Can you work these out from the model? Positions are in its coordinate system, mm. Coordinates: 2 decimals unless noted, no trailing zeros. Order: outer loops, then holes, each group sorted by start corner. A loop starts at its lowest first (then second) coordinate and runs counter-clockwise, first axis right, second up. Notation, with made-up numbers: (-12, -39.5) -> (28, -39.5) arc R22 cw to (28, -18.5) -> close; hole circle Ø5 at (-16, -15). An arc over 180 degrees is marked (long way). Answer in a Markdown table with one row per item.
```python
from build123d import *

# Parameters (mm, degrees)
SKETCH_1_W      = 74
SKETCH_1_H      = 105
SKETCH_1_R      = 2.1
EXTRUDE_1_DEPTH = 3
FILLET_1_R      = 5
CHAMFER_1_SIZE  = 1.5


with BuildPart() as part:
    # ｽｹｯﾁ1 → ﾎﾞｽ - 押し出し1 (new body)
    with BuildSketch(Plane.XY):
        Rectangle(SKETCH_1_W, SKETCH_1_H)
        with Locations((-16, 36)):
            Circle(SKETCH_1_R, mode=Mode.SUBTRACT)
        with Locations((16, 36)):
            Circle(SKETCH_1_R, mode=Mode.SUBTRACT)
        with Locations((-16, 4)):
            Circle(SKETCH_1_R, mode=Mode.SUBTRACT)
        with Locations((16, 4)):
            Circle(SKETCH_1_R, mode=Mode.SUBTRACT)
        with Locations((-29.5, 45)):
            Circle(SKETCH_1_R, mode=Mode.SUBTRACT)
        with Locations((-29.5, -45)):
            Circle(SKETCH_1_R, mode=Mode.SUBTRACT)
        with Locations((29.5, 45)):
            Circle(SKETCH_1_R, mode=Mode.SUBTRACT)
        with Locations((29.5, -45)):
            Circle(SKETCH_1_R, mode=Mode.SUBTRACT)
    extrude(amount=EXTRUDE_1_DEPTH)

    # ﾌｨﾚｯﾄ1
    fillet_1_edges = [part.edges().sort_by_distance(p)[0] for p in [
        (37, -52.5, 1.5),
        (-37, -52.5, 1.5),
        (-37, 52.5, 1.5),
        (37, 52.5, 1.5),
    ]]
    fillet(fillet_1_edges, radius=FILLET_1_R)

    # 面取り1
    chamfer_1_edges = [part.edges().sort_by_distance(p)[0] for p in [
        (-18.1, 36, 3),
        (13.9, 36, 3),
        (-18.1, 4, 3),
        (13.9, 4, 3),
    ]]
    chamfer(chamfer_1_edges, length=CHAMFER_1_SIZE)


solid = part.part
```
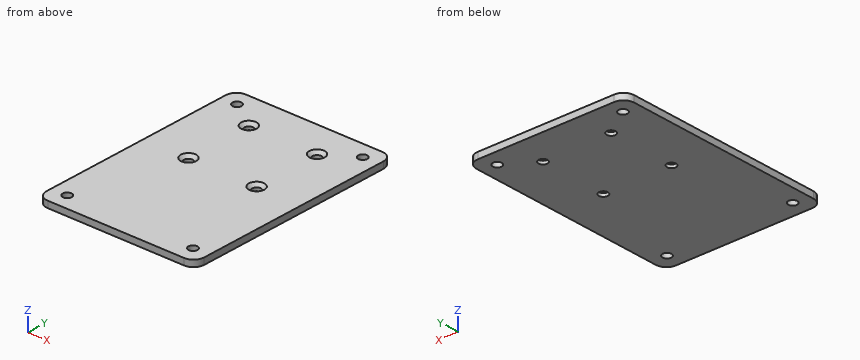
(1) Will this pin go through, and if not, where does the flat tip stop? pin 1 Ø4 at (x, y) = (-16, 36) entering from -Z.
Response values:
| item | result |
|---|---|
| pin 1 | through |
(2) I need wall thicknesses on line 1 (Y direction, x = 29.5, z = 1.4); line 2 (Y direction, x = 18, z = 1.85); line 3 (X direction, y = 44, z = 0.55). Which ranges of each line are inside material? Lowest first, please. Write a range as [from, to].
Response values:
| item | result |
|---|---|
| line 1 | [-52.5, -47.1], [-42.9, 42.9], [47.1, 52.5] |
| line 2 | [-52.5, 2.58], [5.42, 34.58], [37.42, 52.5] |
| line 3 | [-37, -31.35], [-27.65, 27.65], [31.35, 37] |
(3) Suppose I cut it at A-A (z = 1.05). Count the separate pieces of the cut face and the enclosed holes in it, and give its area (3 significant figures).
Response values:
| item | result |
|---|---|
| separate pieces | 1 |
| enclosed holes | 8 |
| area | 7,640 mm2 |
(4) Suppose I cut it at C-C (y = 4). Please give me the cut outline in (x, z).
Response values:
| item | result |
|---|---|
| outline | (-37, 0) -> (-18.1, 0) -> (-18.1, 1.5) -> (-19.6, 3) -> (-37, 3) -> close; (-13.9, 0) -> (13.9, 0) -> (13.9, 1.5) -> (12.4, 3) -> (-12.4, 3) -> (-13.9, 1.5) -> close; (18.1, 0) -> (37, 0) -> (37, 3) -> (19.6, 3) -> (18.1, 1.5) -> close |
(5) Suppose I cut it at B-B (x = 16). Please give me the cut outline in (y, z).
Response values:
| item | result |
|---|---|
| outline | (-52.5, 0) -> (1.9, 0) -> (1.9, 1.5) -> (0.4, 3) -> (-52.5, 3) -> close; (6.1, 0) -> (33.9, 0) -> (33.9, 1.5) -> (32.4, 3) -> (7.6, 3) -> (6.1, 1.5) -> close; (38.1, 0) -> (52.5, 0) -> (52.5, 3) -> (39.6, 3) -> (38.1, 1.5) -> close |
(6) Suppose I cut it at D-D (x = 29.5). Please give me the cut outline in (y, z), and give its area (3 significant figures).
Response values:
| item | result |
|---|---|
| outline | (-52.5, 0) -> (-47.1, 0) -> (-47.1, 3) -> (-52.5, 3) -> close; (-42.9, 0) -> (42.9, 0) -> (42.9, 3) -> (-42.9, 3) -> close; (47.1, 0) -> (52.5, 0) -> (52.5, 3) -> (47.1, 3) -> close |
| area | 290 mm2 |
